Design review of the part shown in the three views and the two pictorial views. Dimensions are in mm from the part's minimum x, y and z. Coordinates: 2 decimals unless noted, no trailing zeros. Loops run counter-clockwise (first coordinate to the right, second up) from the corner with the lowest first, then second, coordinate; pieces in that order, holes last. Notation, with made-up numbers: (-3.5, 4) -> (45.5, 4) arc R10 cw to (45.5, 10) -> close; hole circle Ø5 at (-30, 83.25). An arc over 180 degrees is marked (long way). Use CSV: the item, a comma, the result in double quotes.
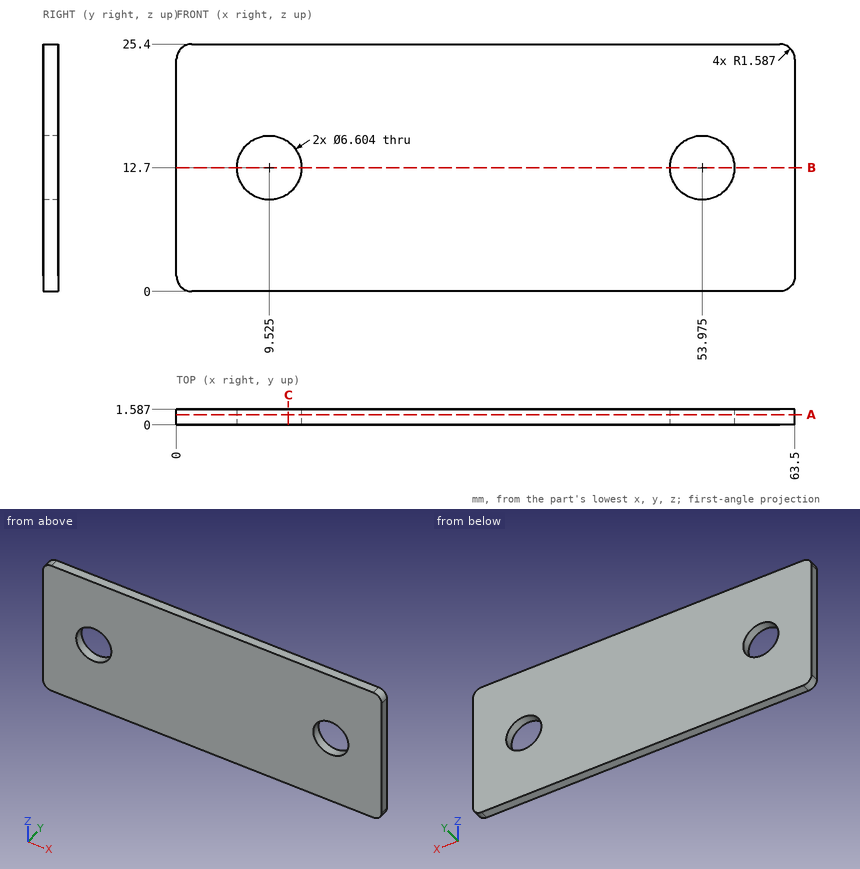
Item 1: To check wall thickness, follow line 1 along X through (y, z) = (0.4, 15.5) (1 decimal); line 2 along X through (y, z) = (1.05, 11.5); line 3 along X through (y, z) = (1.35, 24). State the ranges of each line that lie inside material, in increasing order.
Checked values:
line 1,"0 to 7.8, 11.3 to 52.2, 55.7 to 63.5"
line 2,"0 to 6.45, 12.6 to 50.9, 57.05 to 63.5"
line 3,"0.01 to 63.49"
Item 2: Clearance check with a flat-ended pin moving along its axis: pin 1 (3 mm diameter, centred on x = 23, z = 12.5, fed in from -Y). State where the tip first meets the part, or that it passes through.
Checked values:
pin 1,"y = 0"
Item 3: Add section B-B (z = 12.7). Give the boundary of the cut face in (x, y).
Checked values:
outline,"(0, 0) -> (6.22, 0) -> (6.22, 1.59) -> (0, 1.59) -> close; (12.83, 0) -> (50.67, 0) -> (50.67, 1.59) -> (12.83, 1.59) -> close; (57.28, 0) -> (63.5, 0) -> (63.5, 1.59) -> (57.28, 1.59) -> close"
Item 4: Add section C-C (x = 11.5). Give the boundary of the cut face in (y, z).
Checked values:
outline,"(0, 0) -> (1.59, 0) -> (1.59, 10.05) -> (0, 10.05) -> close; (0, 15.35) -> (1.59, 15.35) -> (1.59, 25.4) -> (0, 25.4) -> close"
Item 5: Add section A-A (y = 1.05). Give the boundary of the cut face in (x, z) (1 decimal).
Checked values:
outline,"(0, 1.6) arc R1.6 ccw to (1.6, 0) -> (61.9, 0) arc R1.6 ccw to (63.5, 1.6) -> (63.5, 23.8) arc R1.6 ccw to (61.9, 25.4) -> (1.6, 25.4) arc R1.6 ccw to (0, 23.8) -> close; hole circle Ø6.6 at (9.5, 12.7); hole circle Ø6.6 at (54, 12.7)"
